```python
from build123d import *

# Parameters (mm, degrees)
SKETCH1_R           = 3.6
BOSS_EXTRUDE1_DEPTH = 1.5
SKETCH2_R           = 1.6
SKETCH2_R_2         = 8.25
SKETCH2_W           = 22
SKETCH2_H           = 22
SKETCH2_W_2         = 30
CUT_EXTRUDE1_DEPTH  = 278.202994212


with BuildPart() as part:
    # Sketch1 → Boss-Extrude1 (new body)
    with BuildSketch(Plane(origin=(0, 0, 0), x_dir=(1, 0, 0), z_dir=(0, 1, 0))):
        with BuildLine():
            Line((235, -74.5), (-235, -74.5))
            ThreePointArc((-235, -74.5), (-257.627416998, -65.127416998), (-267, -42.5))
            Line((-267, -42.5), (-267, 42.5))
            ThreePointArc((-267, 42.5), (-257.627416998, 65.127416998), (-235, 74.5))
            Line((-235, 74.5), (235, 74.5))
            ThreePointArc((235, 74.5), (257.627416998, 65.127416998), (267, 42.5))
            Line((267, 42.5), (267, -42.5))
            ThreePointArc((267, -42.5), (257.627416998, -65.127416998), (235, -74.5))
        make_face()
        with Locations(Location((-259, 0, 0), (0, 0, 270))):
            Circle(SKETCH1_R, mode=Mode.SUBTRACT)
        with Locations(Location((259, 0, 0), (0, 0, 270))):
            Circle(SKETCH1_R, mode=Mode.SUBTRACT)
        with Locations(Location((-220, 66.5, 0), (0, 0, 270))):
            Circle(SKETCH1_R, mode=Mode.SUBTRACT)
        with Locations(Location((-110, 66.5, 0), (0, 0, 270))):
            Circle(SKETCH1_R, mode=Mode.SUBTRACT)
        with Locations(Location((0, 66.5, 0), (0, 0, 270))):
            Circle(SKETCH1_R, mode=Mode.SUBTRACT)
        with Locations(Location((110, 66.5, 0), (0, 0, 270))):
            Circle(SKETCH1_R, mode=Mode.SUBTRACT)
        with Locations(Location((220, 66.5, 0), (0, 0, 270))):
            Circle(SKETCH1_R, mode=Mode.SUBTRACT)
        with Locations(Location((220, -66.5, 0), (0, 0, 90))):
            Circle(SKETCH1_R, mode=Mode.SUBTRACT)
        with Locations(Location((110, -66.5, 0), (0, 0, 90))):
            Circle(SKETCH1_R, mode=Mode.SUBTRACT)
        with Locations(Location((0, -66.5, 0), (0, 0, 90))):
            Circle(SKETCH1_R, mode=Mode.SUBTRACT)
        with Locations(Location((-110, -66.5, 0), (0, 0, 90))):
            Circle(SKETCH1_R, mode=Mode.SUBTRACT)
        with Locations(Location((-220, -66.5, 0), (0, 0, 90))):
            Circle(SKETCH1_R, mode=Mode.SUBTRACT)
    extrude(amount=BOSS_EXTRUDE1_DEPTH)

    # Sketch2 → Cut-Extrude1 (cut, through all)
    with BuildSketch(Plane(origin=(0, 0, 0), x_dir=(1, 0, 0), z_dir=(0, 1, 0))):
        with Locations(Location((-210, 10, 0), (0, 0, 270))):
            Circle(SKETCH2_R)
        with Locations(Location((-210, 40, 0), (0, 0, 270))):
            Circle(SKETCH2_R)
        with Locations(Location((-100, 0, 0), (0, 0, 270))):
            Circle(SKETCH2_R_2)
        with Locations((-210, 25)):
            Rectangle(SKETCH2_W, SKETCH2_H)
        with BuildLine():
            Line((-151.75, 15.638181697), (-148.25, 15.638181697))
            Line((-148.25, 15.638181697), (-148.25, 13.638181697))
            ThreePointArc((-148.25, 13.638181697), (-150, -13.75), (-151.75, 13.638181697))
            Line((-151.75, 13.638181697), (-151.75, 15.638181697))
        make_face()
        with Locations((-210, -25)):
            Rectangle(SKETCH2_W_2, SKETCH2_H)
        with BuildLine():
            Line((-31.5, 30.5), (-48.5, 30.5))
            ThreePointArc((-48.5, 30.5), (-49.560660172, 30.060660172), (-50, 29))
            Line((-50, 29), (-50, 26.5))
            Line((-50, 26.5), (-52.6, 26.5))
            ThreePointArc((-52.6, 26.5), (-54.1, 25), (-52.6, 23.5))
            Line((-52.6, 23.5), (-50, 23.5))
            Line((-50, 23.5), (-50, 21))
            ThreePointArc((-50, 21), (-49.560660172, 19.939339828), (-48.5, 19.5))
            Line((-48.5, 19.5), (-31.5, 19.5))
            ThreePointArc((-31.5, 19.5), (-30.439339828, 19.939339828), (-30, 21))
            Line((-30, 21), (-30, 23.5))
            Line((-30, 23.5), (-27.4, 23.5))
            ThreePointArc((-27.4, 23.5), (-25.9, 25), (-27.4, 26.5))
            Line((-27.4, 26.5), (-30, 26.5))
            Line((-30, 26.5), (-30, 29))
            ThreePointArc((-30, 29), (-30.439339828, 30.060660172), (-31.5, 30.5))
        make_face()
        with BuildLine():
            Line((-31.5, -19.5), (-48.5, -19.5))
            ThreePointArc((-48.5, -19.5), (-49.560660172, -19.939339828), (-50, -21))
            Line((-50, -21), (-50, -23.5))
            Line((-50, -23.5), (-52.6, -23.5))
            ThreePointArc((-52.6, -23.5), (-54.1, -25), (-52.6, -26.5))
            Line((-52.6, -26.5), (-50, -26.5))
            Line((-50, -26.5), (-50, -29))
            ThreePointArc((-50, -29), (-49.560660172, -30.060660172), (-48.5, -30.5))
            Line((-48.5, -30.5), (-31.5, -30.5))
            ThreePointArc((-31.5, -30.5), (-30.439339828, -30.060660172), (-30, -29))
            Line((-30, -29), (-30, -26.5))
            Line((-30, -26.5), (-27.4, -26.5))
            ThreePointArc((-27.4, -26.5), (-25.9, -25), (-27.4, -23.5))
            Line((-27.4, -23.5), (-30, -23.5))
            Line((-30, -23.5), (-30, -21))
            ThreePointArc((-30, -21), (-30.439339828, -19.939339828), (-31.5, -19.5))
        make_face()
    extrude(amount=CUT_EXTRUDE1_DEPTH, mode=Mode.SUBTRACT)


solid = part.part
```
Geometry: final body of the model. Coordinates: model frame, mm. Coordinates: 2 decimals unless noted, no trailing zeros. Answer as CSV lines item,"result". Start each with the question number.
Q1. Cut plane A-A on y = 0.9. Count the separate pieces of the cut face and the enclosed holes in it, then the cut area to 3 significant figures.
Q2. Line query: line 1 (Z direction, x = -220, y = 1); line 2 (Z direction, x = -210, y = 1.05); line 3 (X direction, y = 0.8, z = 0). Output: solid intervals per line, ascending. Write a range as from..to.
Q3. Pin query (flat end, axial travel): P1, Ø8, axis at x = 183, z = 56, coming from the -Y side. Return the tip coordinate at first contact, or that it passes through.
Q4. Mould query, pull axis X, two halves, no side actions, for faces 1 (the cylindrical face through (-149.42, 0.74, 13.738)), 2 (the cylindrical face through (-108.054, 0.74, -1.788)), 3 (the cylindrical face through (-257.87, 0.74, -64.88)), 4 (the flat face through (4, 1.5, -1)). Classes: released by +X, released by -X, zero draft, split by the parting line, or undercut.
Findings below:
1,separate pieces,"1"
1,enclosed holes,"20"
1,area,"75,700 mm2"
2,line 1,"z = -74.5..-70.1, -62.9..-36, -14..14, 36..62.9, 70.1..74.5"
2,line 2,"z = -74.5..-41.6, -38.4..-36, -14..-11.6, -8.4..14, 36..74.5"
2,line 3,"x = -267..-262.6, -255.4..-163.75, -136.25..-108.25, -91.75..255.4, 262.6..267"
3,P1,"stops at y = 0"
4,face 1,"undercut"
4,face 2,"undercut"
4,face 3,"released by -X"
4,face 4,"zero draft"
